CAD build for the part. Positions are in the model's coordinates, mm. A direction names the side the tool comes from. Give positions to 0.01 mm unless a question says otherwise; leave off trailing zeros. Loops run counter-clockwise (first coordinate to the right, second up) from the corner with the lowest first, then second, coordinate; pieces in that order, holes last. Notation, with made-up numbers: (20, -1) -> (41, -1) arc R9 ccw to (41, 6) -> close; hole circle Ø5 at (-3, 22). An arc over 180 degrees is marked (long way). Use one line per item in the form item = value.
```python
from build123d import *

# Parameters (mm, degrees)
F0_W        = 25
F0_H        = 20
F1_DEPTH    = 5
F3_DEPTH    = 0.75
F4_T1_DEPTH = 1.5
F4_T3_DEPTH = 11.5
F5_SIZE     = 1.99999


# Not quite as in the source:
# - a fillet or chamfer that OpenCascade refuses, or shapes differently, is made with other operations: its cross-section is extruded or revolved along the edge and cut away or added
# - a fillet or chamfer is up to 0.001 mm smaller than in the source, because OpenCascade refuses the exact size


with BuildPart() as f1:
    # F0 (on Top) → F1 (new body)
    with BuildSketch(Plane.XY):
        Rectangle(F0_W, F0_H)
    extrude(amount=-F1_DEPTH)

    # F2 (on Right) → F3 (join, symmetric)
    with BuildSketch(Plane.YZ):
        Polygon((-6, 4), (-6, 0), (-5, 0), (-5, 3), (5, 3), (5, 0), (6, 0), (6, 4), align=None)
    extrude(amount=F3_DEPTH, both=True)

    # F4: fillet of radius 2 on 8 edges, made by hand

    # F4_s2 → F4_t1 (join)
    with BuildSketch(Plane.YZ.offset(-0.75)):
        with BuildLine():
            ThreePointArc((-3, 0), (-4.4142135624, 0.5857864376), (-5, 2))
            Line((-5, 2), (-5, 0))
            Line((-5, 0), (-3, 0))
        make_face()
        with BuildLine():
            ThreePointArc((3, 0), (4.4142135624, 0.5857864376), (5, 2))
            Line((5, 2), (5, 0))
            Line((5, 0), (3, 0))
        make_face()
        with BuildLine():
            ThreePointArc((-8, 0), (-6.5857864376, 0.5857864376), (-6, 2))
            Line((-6, 2), (-6, 0))
            Line((-6, 0), (-8, 0))
        make_face()
        with BuildLine():
            ThreePointArc((8, 0), (6.5857864376, 0.5857864376), (6, 2))
            Line((6, 2), (6, 0))
            Line((6, 0), (8, 0))
        make_face()
        with BuildLine():
            ThreePointArc((-5, 1), (-4.4142135624, 2.4142135624), (-3, 3))
            Line((-3, 3), (-5, 3))
            Line((-5, 3), (-5, 1))
        make_face()
        with BuildLine():
            ThreePointArc((5, 1), (4.4142135624, 2.4142135624), (3, 3))
            Line((3, 3), (5, 3))
            Line((5, 3), (5, 1))
        make_face()
    extrude(amount=F4_T1_DEPTH)

    # F4_s4 → F4_t3 (cut)
    with BuildSketch(Plane.YZ.offset(-5.75)):
        with BuildLine():
            ThreePointArc((-4, 4), (-5.4142135624, 3.4142135624), (-6, 2))
            Line((-6, 2), (-6, 4))
            Line((-6, 4), (-4, 4))
        make_face()
        with BuildLine():
            ThreePointArc((6, 2), (5.4142135624, 3.4142135624), (4, 4))
            Line((4, 4), (6, 4))
            Line((6, 4), (6, 2))
        make_face()
    extrude(amount=F4_T3_DEPTH, mode=Mode.SUBTRACT)

    # F5 (size 2 in the source; OpenCascade refuses exactly that, so slightly less here)
    f5_edges = [f1.edges().sort_by_distance(p)[0] for p in [
        (12.5, 0, 0),
        (0, -10, 0),
        (0, 10, 0),
        (-12.5, 0, 0),
    ]]
    chamfer(f5_edges, length=F5_SIZE)


solid = f1.part
```
1. Drop flat-ended pins along their axis: P1, Ø3, axis at y = 0, z = 1, coming from the -X side; P2, Ø1.5, axis at y = 5.5, z = -0.5, coming from the -X side; P3, Ø1.5, axis at y = -2.5, z = 0.5, coming from the -X side; P4, Ø5, axis at y = -6.5, z = -1.5, coming from the -X side. Give the stop position or say it passes through.
Result sheet:
P1 = -11
P2 = -11.75
P3 = -10.75
P4 = -12.5
2. Mould opens along Z. For faces 4 (the flat face through (0, 10, -3)), 5 (the flat face through (-11.5, -0.1, -1)), 6 (the cylindrical face through (0, 4.2, 2.6)) say: pulls with the +Z half, pulls with the -Z half, needs draft (parallel to the pull), parting line crosses it, or undercut.
Result sheet:
face_4 = needs draft
face_5 = pulls with the +Z half
face_6 = undercut
3. Tool access for faces 1 (the flat face through (-0.75, 0, 3.2)), 2 (the flat face through (0.75, 0, 3.2)), 3 (the flat face through (0, 0, 3)): list every direction of +Z, -Z, +X, -X, +Y, -Y with a clear straight run to the whole face (end or side of a thin tool).
Result sheet:
face_1 = +Z, -X, +Y, -Y
face_2 = +Z, +X, +Y, -Y
face_3 = +X, -X
4. Drill centre lines: line 1 (Z direction, x = 6.5, y = -3.75); line 2 (X direction, y = -2.5, z = 3.25); line 3 (Y direction, x = -0.5, z = 1). Where is each one in solid material? Low to high.
Result sheet:
line_1 = -5 to 0
line_2 = -0.75 to 0.75
line_3 = -6.27 to -4.73, 4.73 to 6.27
5. Cut at C-C, the plane y = 6.75. Write the cut outline in (x, z), then the cut area to 3 significant figures.
Result sheet:
outline = (-12.5, -5) -> (12.5, -5) -> (12.5, -2) -> (10.5, 0) -> (0.75, 0) -> (0.75, 0.44) -> (-0.75, 0.44) -> (-0.75, 0) -> (-10.5, 0) -> (-12.5, -2) -> close
area = 122 mm^2
6. Cut at B-B, the plane y = 1.5. Write the cut outline in (x, z).
Result sheet:
outline = (-12.5, -5) -> (12.5, -5) -> (12.5, -2) -> (10.5, 0) -> (-10.5, 0) -> (-12.5, -2) -> close; (-0.75, 3) -> (0.75, 3) -> (0.75, 4) -> (-0.75, 4) -> close
7. Cut at D-D, the plane z = -1. Write the cut outline in (x, y), then the cut area to 3 significant figures.
Result sheet:
outline = (-11.5, -9) -> (11.5, -9) -> (11.5, 9) -> (-11.5, 9) -> close
area = 414 mm^2
